Input: part model. Units: mm. Frame: model coordinates. Give positions to 0.01 mm unless a question says otherwise; leave off trailing zeros. Order: outer loops, then holes, each group sorted by start corner. A loop starts at its lowest first (then second) coordinate and runs counter-clockwise, first axis right, second up. Notation, with made-up numbers: M 10,80.25 L 23,80.25 A30 cw 23,113.25 Z; hole C 2.5,8.5 d1. An arc over 180 degrees is marked long. Use a Markdown table: item, result.
from build123d import *

# Parameters (mm, degrees)
SKETCH1_R           = 86.9315
BOSS_EXTRUDE1_DEPTH = 2.54
SKETCH3_W           = 104.14
SKETCH3_H           = 104.14
CUT_EXTRUDE2_DEPTH  = 2.54
SKETCH4_R           = 3.175
CUT_EXTRUDE3_DEPTH  = 2.54
SKETCH5_R           = 12.7
CUT_EXTRUDE4_DEPTH  = 123.965942376
CIRPATTERN1_COUNT   = 4


with BuildPart() as part:
    # Sketch1 → Boss-Extrude1 (new body)
    with BuildSketch(Plane(origin=(0, 0, 0), x_dir=(1, 0, 0), z_dir=(0, 1, 0))):
        with Locations(Location((0, 0, 0), (0, 0, 270))):
            Circle(SKETCH1_R)
    extrude(amount=BOSS_EXTRUDE1_DEPTH)

    # Sketch3 → Cut-Extrude2 (cut)
    with BuildSketch(Plane(origin=(0, 2.54, 0), x_dir=(1, 0, 0), z_dir=(0, 1, 0))):
        Rectangle(SKETCH3_W, SKETCH3_H)
    extrude(amount=-CUT_EXTRUDE2_DEPTH, mode=Mode.SUBTRACT)

    # Sketch4 → Cut-Extrude3 (cut)
    with BuildSketch(Plane(origin=(0, 2.54, 0), x_dir=(1, 0, 0), z_dir=(0, 1, 0))):
        with Locations(Location((-32.385, -69.50075, 0), (0, 0, 270))):
            Circle(SKETCH4_R)
        with Locations(Location((-69.50075, -32.385, 0), (0, 0, 270))):
            Circle(SKETCH4_R)
        with Locations(Location((69.50075, 32.385, 0), (0, 0, 270))):
            Circle(SKETCH4_R)
        with Locations(Location((-69.50075, 32.385, 0), (0, 0, 90))):
            Circle(SKETCH4_R)
        with Locations(Location((-32.385, 69.50075, 0), (0, 0, 270))):
            Circle(SKETCH4_R)
        with Locations(Location((32.385, 69.50075, 0), (0, 0, 90))):
            Circle(SKETCH4_R)
        with Locations(Location((69.50075, -32.385, 0), (0, 0, 90))):
            Circle(SKETCH4_R)
        with Locations(Location((32.385, -69.50075, 0), (0, 0, 270))):
            Circle(SKETCH4_R)
    extrude(amount=-CUT_EXTRUDE3_DEPTH, mode=Mode.SUBTRACT)

    # Sketch5 → Cut-Extrude4 (cut, through all)
    with BuildSketch(Plane(origin=(0, 2.54, 0), x_dir=(1, 0, 0), z_dir=(0, 1, 0))):
        with Locations(Location((-69.738430692, 0, 0), (0, 0, 270))):
            Circle(SKETCH5_R)
    cut_extrude4 = extrude(amount=-CUT_EXTRUDE4_DEPTH, mode=Mode.SUBTRACT)

    # CirPattern1: Cut-Extrude4 ×4 about axis
    cirpattern1_axis = Axis((0, 0, 0), (0, 1, 0))
    for i in range(1, CIRPATTERN1_COUNT):
        add(cut_extrude4.rotate(cirpattern1_axis, i * 360 / CIRPATTERN1_COUNT), mode=Mode.SUBTRACT)


solid = part.part
1) First-contact query: pin 1 Ø0.8 at (x, y) = (-22, 1) entering from +Z; pin 2 Ø10 at (x, z) = (-69.5, 32.38) entering from -Y; pin 3 Ø1 at (x, y) = (-16.5, 0.5) entering from +Z; pin 4 Ø4 at (x, z) = (32.38, -69.5) entering from +Y. Flat tips, straight axial feed; report the tip coordinate or a pass-through.
Response values:
| item | result |
|---|---|
| pin 1 | stops at z = 84.21 |
| pin 2 | stops at y = 0 |
| pin 3 | stops at z = 85.45 |
| pin 4 | passes through |
2) Cut plane C-C on z = -27. Return loops of the section in (x, y).
Response values:
| item | result |
|---|---|
| outline | M -82.63,0 L -52.07,0 L -52.07,2.54 L -82.63,2.54 Z; M 52.07,0 L 82.63,0 L 82.63,2.54 L 52.07,2.54 Z |
3) Material intervals for line 1 (Z direction, x = -1, y = 0.2); line 2 (X direction, y = 1.8, z = 0); line 3 (Z direction, x = 70.5, y = 1.1), sorted ascending. Write a range as from..to.
Response values:
| item | result |
|---|---|
| line 1 | z = -86.93..-82.4, -57.08..-52.07, 52.07..57.08, 82.4..86.93 |
| line 2 | x = -86.93..-82.44, -57.04..-52.07, 52.07..57.04, 82.44..86.93 |
| line 3 | z = -50.86..-35.4, -29.37..-12.68, 12.68..29.37, 35.4..50.86 |
4) Cut plane B-B on z = 0. Return loops of the section in (x, y), and give its area (3 significant figures).
Response values:
| item | result |
|---|---|
| outline | M -86.93,0 L -82.44,0 L -82.44,2.54 L -86.93,2.54 Z; M -57.04,0 L -52.07,0 L -52.07,2.54 L -57.04,2.54 Z; M 52.07,0 L 57.04,0 L 57.04,2.54 L 52.07,2.54 Z; M 82.44,0 L 86.93,0 L 86.93,2.54 L 82.44,2.54 Z |
| area | 48.1 mm² |
5) Cut plane A-A on x = 0. Return loops of the section in (y, z), and give its area (3 significant figures).
Response values:
| item | result |
|---|---|
| outline | M 0,-86.93 L 2.54,-86.93 L 2.54,-82.44 L 0,-82.44 Z; M 0,-57.04 L 2.54,-57.04 L 2.54,-52.07 L 0,-52.07 Z; M 0,52.07 L 2.54,52.07 L 2.54,57.04 L 0,57.04 Z; M 0,82.44 L 2.54,82.44 L 2.54,86.93 L 0,86.93 Z |
| area | 48.1 mm² |
6) Mould query, pull axis X, two halves, no side actions, for faces 1 (the face through (26.112, 1.252, 82.917)), 2 (the face through (72.18, 1.29, -30.68)), 3 (the face through (-56.7, 2.54, -1.2)). Classes: released by +X, released by -X, zero draft, split by the parting line, or undercut.
Response values:
| item | result |
|---|---|
| face 1 | split by the parting line |
| face 2 | undercut |
| face 3 | zero draft |
7) Cut plane D-D on y = 1. State how many separate pieces and enclosed holes the cut face has, and give its area (3 significant figures).
Response values:
| item | result |
|---|---|
| separate pieces | 1 |
| enclosed holes | 13 |
| area | 10,600 mm² |
